Input: dimensioned drawing with shaded views. Units: mm. Origin: part minimum x, y, z. Coordinates: 2 decimals unless noted, no trailing zeros. Write each loop counter-clockwise with the first axis right and the second up, starting at its lowest first coordinate (ties: lowest second). Pieces come first, ordered by that corner, then holes. Notation, with made-up numbers: (61.25, 10.25) - (71.25, 10.25) arc R11 ccw to (71.25, 17.25) - close; hole circle Ø3 at (39.25, -18). An arc over 180 degrees is marked (long way). One line per question, with ' | ' between items.
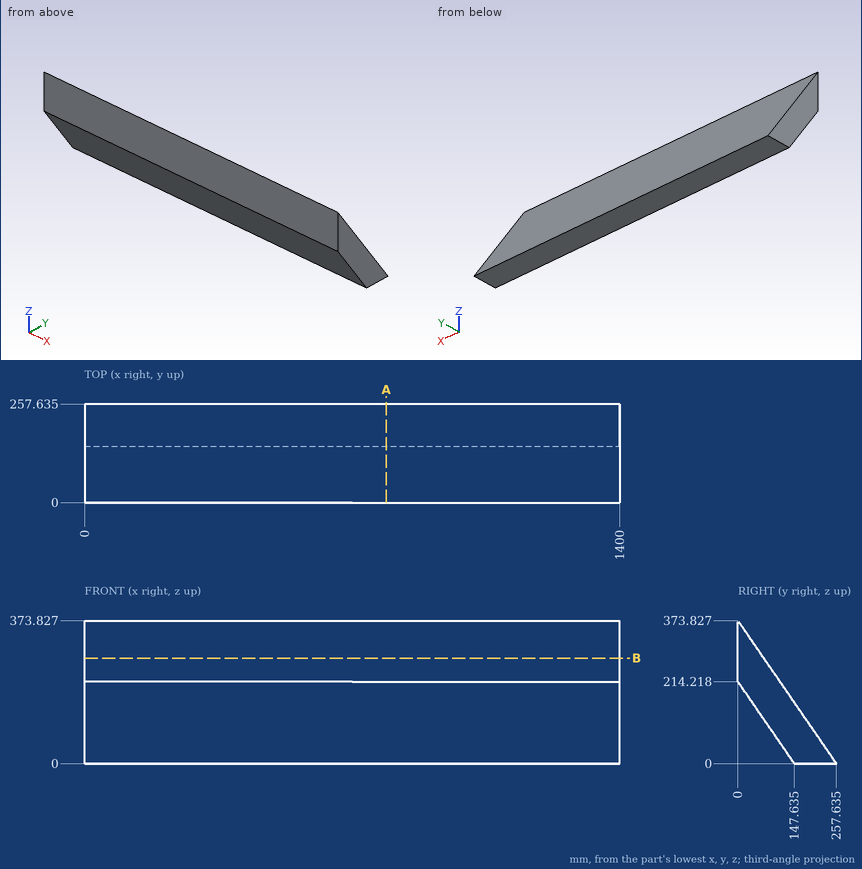
Item 1: Pin query (flat end, axial travel): pin 1 Ø5 at (x, y) = (613, 57.5) entering from -Z; pin 2 Ø10 at (x, y) = (273, 189) entering from +Z (1 decimal); pin 3 Ø2 at (x, y) = (1061, 64) entering from -Z (1 decimal). Return the tip coordinate at first contact, or that it passes through.
Check sheet entries:
pin 1: z = 127.16 | pin 2: z = 106.8 | pin 3: z = 119.9
Item 2: Ray query, line 1 along Y through (x, z) = (614, 310.5) (1 decimal); line 2 along Y through (x, z) = (122, 167.5); line 3 along Z through (x, y) = (272.5, 197.5) (1 decimal). Return the intervals inside material, ascending. Write a range as [from, to].
Check sheet entries:
line 1: [0, 43.6] | line 2: [32.2, 142.2] | line 3: [0, 87.3]
Item 3: Cut plane A-A on x = 789. Return loops of the section in (y, z) (1 decimal).
Check sheet entries:
outline: (0, 214.2) - (147.6, 0) - (257.6, 0) - (0, 373.8) - close
Item 4: Cut plane B-B on z = 275.5. Return loops of the section in (x, y) (1 decimal), and give its area (3 significant figures).
Check sheet entries:
outline: (0, 0) - (1400, 0) - (1400, 67.8) - (0, 67.8) - close | area: 94,900 mm²
